```python
from build123d import *

# Parameters (mm, degrees)
SKETCH1_W           = 300
SKETCH1_H           = 450
BOSS_EXTRUDE1_DEPTH = 5
SKETCH2_R           = 2
CUT_EXTRUDE1_DEPTH  = 271.462566726
FILLET2_R           = 10
FILLET1_R           = 1
SKETCH4_W           = 10
SKETCH4_H           = 410
CUT_EXTRUDE3_DEPTH  = 0.5


with BuildPart() as part:
    # Sketch1 → Boss-Extrude1 (new body)
    with BuildSketch(Plane(origin=(0, 0, 0), x_dir=(1, 0, 0), z_dir=(0, 1, 0))):
        Rectangle(SKETCH1_W, SKETCH1_H)
    extrude(amount=BOSS_EXTRUDE1_DEPTH)

    # Sketch2 → Cut-Extrude1 (cut, through all)
    with BuildSketch(Plane(origin=(0, 5, 0), x_dir=(1, 0, 0), z_dir=(0, 1, 0))):
        with Locations(Location((-140, 0, 0), (0, 0, 270))):
            Circle(SKETCH2_R)
        with Locations(Location((-140, 112.5, 0), (0, 0, 270))):
            Circle(SKETCH2_R)
        with Locations(Location((-140, -112.5, 0), (0, 0, 270))):
            Circle(SKETCH2_R)
        with Locations(Location((-140, 169.5, 0), (0, 0, 270))):
            Circle(SKETCH2_R)
        with Locations(Location((-140, -168.5, 0), (0, 0, 270))):
            Circle(SKETCH2_R)
    extrude(amount=-CUT_EXTRUDE1_DEPTH, mode=Mode.SUBTRACT)

    # Fillet2
    fillet2_edges = [part.edges().sort_by_distance(p)[0] for p in [
        (150, 2.5, 225),
        (-150, 2.5, 225),
        (-150, 2.5, -225),
        (150, 2.5, -225),
    ]]
    fillet(fillet2_edges, radius=FILLET2_R)

    # Fillet1
    fillet1_edges = [part.edges().sort_by_distance(p)[0] for p in [
        (-150, 5, 0),
        (0, 5, -225),
        (150, 5, 0),
        (0, 5, 225),
        (-147.071067812, 5, 222.071067812),
        (147.071067812, 5, 222.071067812),
        (147.071067812, 5, -222.071067812),
        (-147.071067812, 5, -222.071067812),
    ]]
    fillet(fillet1_edges, radius=FILLET1_R)

    # Sketch4 → Cut-Extrude3 (cut)
    with BuildSketch(Plane.XZ):
        with Locations((20, 0)):
            Rectangle(SKETCH4_W, SKETCH4_H)
        Rectangle(SKETCH4_W, SKETCH4_H)
        with Locations((40, 0)):
            Rectangle(SKETCH4_W, SKETCH4_H)
        with Locations((60, 0)):
            Rectangle(SKETCH4_W, SKETCH4_H)
        with Locations((80, 0)):
            Rectangle(SKETCH4_W, SKETCH4_H)
        with Locations((100, 0)):
            Rectangle(SKETCH4_W, SKETCH4_H)
        with Locations((-20, 0)):
            Rectangle(SKETCH4_W, SKETCH4_H)
        with Locations((-40, 0)):
            Rectangle(SKETCH4_W, SKETCH4_H)
        with Locations((-60, 0)):
            Rectangle(SKETCH4_W, SKETCH4_H)
        with Locations((-80, 0)):
            Rectangle(SKETCH4_W, SKETCH4_H)
        with Locations((-100, 0)):
            Rectangle(SKETCH4_W, SKETCH4_H)
    extrude(amount=-CUT_EXTRUDE3_DEPTH, mode=Mode.SUBTRACT)


solid = part.part
```
Read the model definition and answer for the solid it produces. Units are mm, in the model's axes. A direction names the side the tool comes from. Give positions to 0.01 mm unless a question says otherwise; leave off trailing zeros.
(1) For faces 4 (the flat face through (60, 0.5, 3)), 5 (the cylindrical face through (-147.15, 2.03, -221.99)), determine the directions among +Z, -Z, +X, -X, +Y, -Y from which every point of the face is accessible in a straight line to the end or side of a thin tool.
(2) Straight lines are drawn through the part: L1, parallel to Z at x = -140, y = 1.45; L2, parallel to Z at x = 101, y = 0.4; L3, parallel to X at y = 3.25, z = -112.5. For each, find the intervals that lie inside material, in ascending order.
(3) For a pull along X with two mould halves and no side action, classify faces 1 (the flat face through (-40, 0.5, 3)), 2 (the cylindrical face through (-147.15, 2.03, 221.99)), 3 (the cylindrical face through (146.99, 2.03, 222.15)) as released by +X, released by -X, zero draft, split by the parting line, or undercut.
(4) Given pin 1 (6.5 mm diameter, centred on x = -140, z = -112.5, fed in from +Y); pin 2 (5 mm diameter, centred on x = 58.5, z = -157.5, fed in from -Y), each flat-ended and moving along its own axis, determine where each tip first touches the part or whether it passes through.
Result sheet:
1. face 4: -Y
1. face 5: -Z, -X, +Y, -Y
2. L1: z = -225 to -171.5, -167.5 to -114.5, -110.5 to -2, 2 to 110.5, 114.5 to 166.5, 170.5 to 225
2. L2: z = -225 to -205, 205 to 225
2. L3: x = -150 to -142, -138 to 150
3. face 1: undercut
3. face 2: released by -X
3. face 3: released by +X
4. pin 1: stops at y = 5
4. pin 2: stops at y = 0.5
